Could you check a few things on this model? Use its own coordinates, in mm. Face numbers are marked on the shaded views. A direction names the side the tool comes from. Coordinates: 2 decimals unless noted, no trailing zeros. Loops run counter-clockwise (first coordinate to the right, second up) from the corner with the lowest first, then second, coordinate; pieces in that order, holes last. Notation, with made-up numbers: (-8.75, 33.25) -> (39.25, 33.25) arc R24 ccw to (39.25, 52.25) -> close; hole circle Ø3 at (87, 67). An arc over 180 degrees is marked (long way). One line per question, with ' | ' between items. Start each with the question number.
(1) Suppose I cut it at B-B (z = 8.5). Please give me the cut outline in (x, y).
(2) Suppose I cut it at D-D (y = 1.3). Please give me the cut outline in (x, z), plus the area to 3 significant figures.
(3) Which directions (+Z, -Z, +X, -X, +Y, -Y) give clear straight access to the entire face, cutting with the end or side of a thin tool? Please do the marked faces 1 and 2.
(4) If we mould it in two halves opening along X, with no side actions, what happens to the marked faces 3, 4 and 5? For each: pulls with the +X half, pulls with the -X half, needs draft (parallel to the pull), parting line crosses it, or undercut.
(5) Suppose I cut it at C-C (x = -14). Please give me the cut outline in (y, z), plus the area to 3 significant figures.
(6) If I drill on line 1 along X through (y, z) = (-0.15, 4.5); line 2 along X through (y, z) = (0.05, 8); line 3 along Z through (x, y) = (-12, -0.3), over which ranges is the centre line in solid material (lowest first)?
(7) I'm going to push a flat-ended pin straight in: pin 1 Ø1.5 at (y, z) = (1, 7.5) entering from -X. Where does the tip first touch, or does it pass through?
(8) Suppose I cut it at A-A (y = 0). Please give me the cut outline in (x, z).
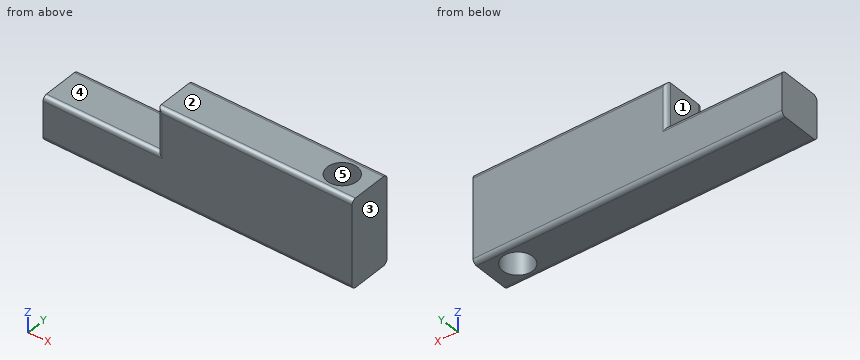
```python
from build123d import *

# Parameters (mm, degrees)
SKETCH1_W            = 35
SKETCH1_H            = 5
BOSS_EXTRUDE1_DEPTH  = 5
SKETCH3_W            = 22
SKETCH3_H            = 5
BOSS_EXTRUDE3_DEPTH  = 5
FILLET1_R            = 0.5
M3_CLEARANCE_HOLE1_D = 3.4


with BuildPart() as part:
    # Sketch1 → Boss-Extrude1 (new body)
    with BuildSketch(Plane.XY):
        Rectangle(SKETCH1_W, SKETCH1_H)
    extrude(amount=BOSS_EXTRUDE1_DEPTH)

    # Sketch3 → Boss-Extrude3 (add)
    with BuildSketch(Plane.XY.offset(5)):
        with Locations((6.5, 0)):
            Rectangle(SKETCH3_W, SKETCH3_H)
    extrude(amount=BOSS_EXTRUDE3_DEPTH)

    # Fillet1
    fillet1_edges = [part.edges().sort_by_distance(p)[0] for p in [
        (-11, 2.5, 5),
        (-4.5, 2.5, 7.5),
        (-4.5, -2.5, 7.5),
        (-11, -2.5, 5),
        (6.5, 2.5, 10),
        (6.5, -2.5, 10),
        (0, -2.5, 0),
        (0, 2.5, 0),
    ]]
    fillet(fillet1_edges, radius=FILLET1_R)

    # M3 Clearance Hole1 (through all)
    with Locations(Plane(origin=(14.415303624, 0, 0), x_dir=(-1, 0, 0), z_dir=(0, 0, -1))):
        with Locations((0, 0)):
            Hole(M3_CLEARANCE_HOLE1_D / 2)


solid = part.part
```
Checks:
1) outline: (-4.5, -2) arc R0.5 ccw to (-4, -2.5) -> (17.5, -2.5) -> (17.5, 2.5) -> (-4, 2.5) arc R0.5 ccw to (-4.5, 2) -> close; hole circle Ø3.4 at (14.42, 0)
2) outline: (-17.5, 0) -> (13.32, 0) -> (13.32, 10) -> (-4.5, 10) -> (-4.5, 5) -> (-17.5, 5) -> close; (15.51, 0) -> (17.5, 0) -> (17.5, 10) -> (15.51, 10) -> close | area: 263 mm^2
3) face 1: +Z, -X, +Y, -Y | face 2: +Z, +X, -X, +Y, -Y
4) face 3: pulls with the +X half | face 4: needs draft | face 5: undercut
5) outline: (-2.5, 0.5) arc R0.5 ccw to (-2, 0) -> (2, 0) arc R0.5 ccw to (2.5, 0.5) -> (2.5, 4.5) arc R0.5 ccw to (2, 5) -> (-2, 5) arc R0.5 ccw to (-2.5, 4.5) -> close | area: 24.8 mm^2
6) line 1: x = -17.5 to 12.72, 16.11 to 17.5 | line 2: x = -4.5 to 12.72, 16.11 to 17.5 | line 3: z = 0 to 5
7) pin 1: stops at x = -4.5
8) outline: (-17.5, 0) -> (12.72, 0) -> (12.72, 10) -> (-4.5, 10) -> (-4.5, 5) -> (-17.5, 5) -> close; (16.12, 0) -> (17.5, 0) -> (17.5, 10) -> (16.12, 10) -> close
